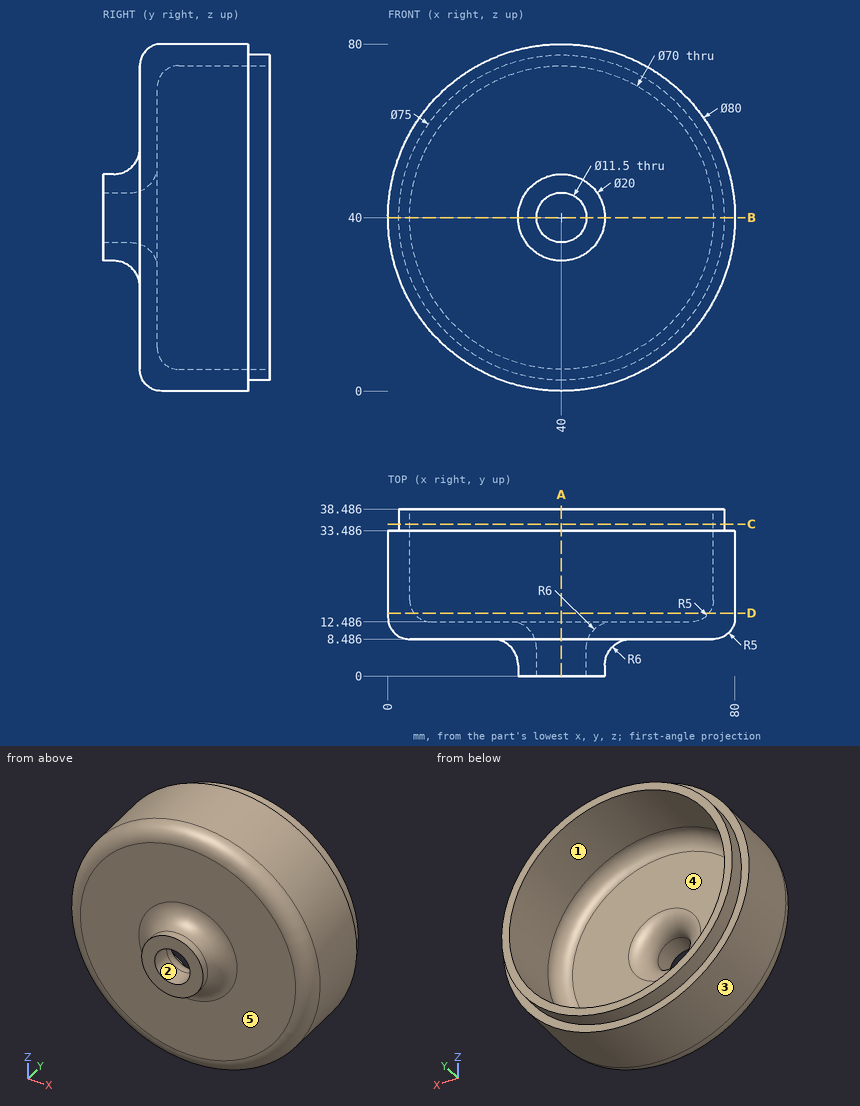
Input: dimensioned drawing with shaded views. Units: mm. Origin: part minimum x, y, z. A direction names the side the tool comes from. Give positions to 0.01 mm unless a question says otherwise; leave off trailing zeros. Loops run counter-clockwise (first coordinate to the right, second up) from the corner with the lowest first, then second, coordinate; pieces in that order, holes last. Notation, with made-up numbers: M 45.25,-13.5 L 102.25,-13.5 A23 cw 102.25,12.5 Z; hole C 64,25 d10. An arc over 180 degrees is marked long. Put each result on its own line as item: value. Start each with the question number.
1) Cut plane A-A (x = 40). Output: boundary loops of the cut face in (y, z), then the cut area to 3 significant figures.
2) Access query for the marked faces 1 and 2. Directions: +Z, -Z, +X, -X, +Y, -Y. A direction counts if a zero-diameter tool reaches every point of the face in a straight line with its end or side. Return the directions, or none.
3) Contact query for flat-ended pins moving along their axis: pin 1 (8 mm diameter, centred on y = 5.5, z = 14.5, fed in from -X); pin 2 (5 mm diameter, centred on x = 8.5, z = 37, fed in from +Y) (1 decimal); pin 3 (2 mm diameter, centred on x = 71, y = 22, fed in from +Z). Output: stop coordinate, or through.
4) Pull-direction query (Z, two-part tool) for the marked faces 3, 4 and 5; classes: pulls with the +Z half, pulls with the -Z half, needs draft (parallel to the pull), parting line crosses it, or undercut.
5) Ray query, line 1 along X through (y, z) = (1.75, 40); line 2 along X through (y, z) = (29.75, 40). Return the intervals inside material, ascending.
6) Cut plane C-C (y = 35). Output: boundary loops of the cut face in (x, z).
7) Cut plane D-D (y = 14.5). Output: boundary loops of the cut face in (x, z).
8) Cut plane B-B (z = 40). Output: boundary loops of the cut face in (x, y), then the cut area to 3 significant figures.
Verdict:
1. outline: M 0,30 L 2.49,30 A6 cw 8.49,24 L 8.49,5 A5 ccw 13.49,0 L 33.49,0 L 33.49,2.5 L 38.49,2.5 L 38.49,5 L 17.49,5 A5 cw 12.49,10 L 12.49,28.25 A6 ccw 6.49,34.25 L 0,34.25 Z; M 0,45.75 L 6.49,45.75 A6 ccw 12.49,51.75 L 12.49,70 A5 cw 17.49,75 L 38.49,75 L 38.49,77.5 L 33.49,77.5 L 33.49,80 L 13.49,80 A5 ccw 8.49,75 L 8.49,56 A6 cw 2.49,50 L 0,50 Z
1. area: 581 mm2
2. face 1: +Y
2. face 2: +Y, -Y
3. pin 1: x = 11.07
3. pin 2: y = 14.7
3. pin 3: z = 66.46
4. face 3: parting line crosses it
4. face 4: undercut
4. face 5: needs draft
5. line 1: 30 to 34.25, 45.75 to 50
5. line 2: 0 to 5, 75 to 80
6. outline: C 40,40 d75; hole C 40,40 d70
7. outline: C 40,40 d80; hole C 40,40 d68.02
8. outline: M 0,13.49 A5 ccw 5,8.49 L 24,8.49 A6 cw 30,2.49 L 30,0 L 34.25,0 L 34.25,6.49 A6 ccw 28.25,12.49 L 10,12.49 A5 cw 5,17.49 L 5,38.49 L 2.5,38.49 L 2.5,33.49 L 0,33.49 Z; M 45.75,0 L 50,0 L 50,2.49 A6 cw 56,8.49 L 75,8.49 A5 ccw 80,13.49 L 80,33.49 L 77.5,33.49 L 77.5,38.49 L 75,38.49 L 75,17.49 A5 cw 70,12.49 L 51.75,12.49 A6 ccw 45.75,6.49 Z
8. area: 581 mm2
